Study the drawing (mm; zero at the part's minimum x, y, z) and answer. A direction names the side the tool comes from. Coordinates: 2 decimals unless noted, no trailing zeros. Write each loop counter-clockwise with the first axis right and the second up, starting at its lowest first coordinate (ties: lowest second). Pieces come first, ordered by that corner, then holes. Notation, with made-up numbers: (-10.75, 73.5) -> (9.25, 73.5) arc R23 ccw to (9.25, 94.5) -> close; hole circle Ø5 at (-27, 38). An arc over 180 degrees is marked (long way). Write item = value, one per line. Start each with the question number.
1) A tool of negligible diameter and unlimited length cuts with its end or side. For the marked faces 1 and 2, from which of +Z, -Z, +X, -X, +Y, -Y can it reach the whole face along a straight path? Write none if from no direction.
2) For a pull along Z with two mould halves and no side action, classify the marked faces 3, 4 and 5 as released by +Z, released by -Z, zero draft, split by the parting line, or undercut.
3) Flat-ended cylindrical pins translate along their axes: pin 1 Ø6.5 at (y, z) = (38.1, 11.11) entering from +X; pin 2 Ø11 at (y, z) = (25.5, 10.5) entering from +X (1 decimal); pin 3 Ø4 at (x, z) = (16.5, 7.5) entering from +Y (1 decimal); pin 4 Ø10 at (x, z) = (6.5, 12) entering from +Y. Find the tip coordinate at first contact, or state that the pin passes through.
4) Section A-A (x = 12.7) is taken. Determine the outline of the cut face in (y, z) (1 decimal).
5) Find the intervals of material crossed by line 1 along Z through (x, y) = (12.7, 2.7) (1 decimal); line 2 along X through (y, z) = (10.5, 17) (1 decimal); line 3 along Z through (x, y) = (3, 14) (1 decimal), in increasing order. Write a range as from..to.
6) Section C-C (z = 12.5) is taken. Count the separate pieces of the cut face and the enclosed holes in it, plus the area to 3 significant figures.
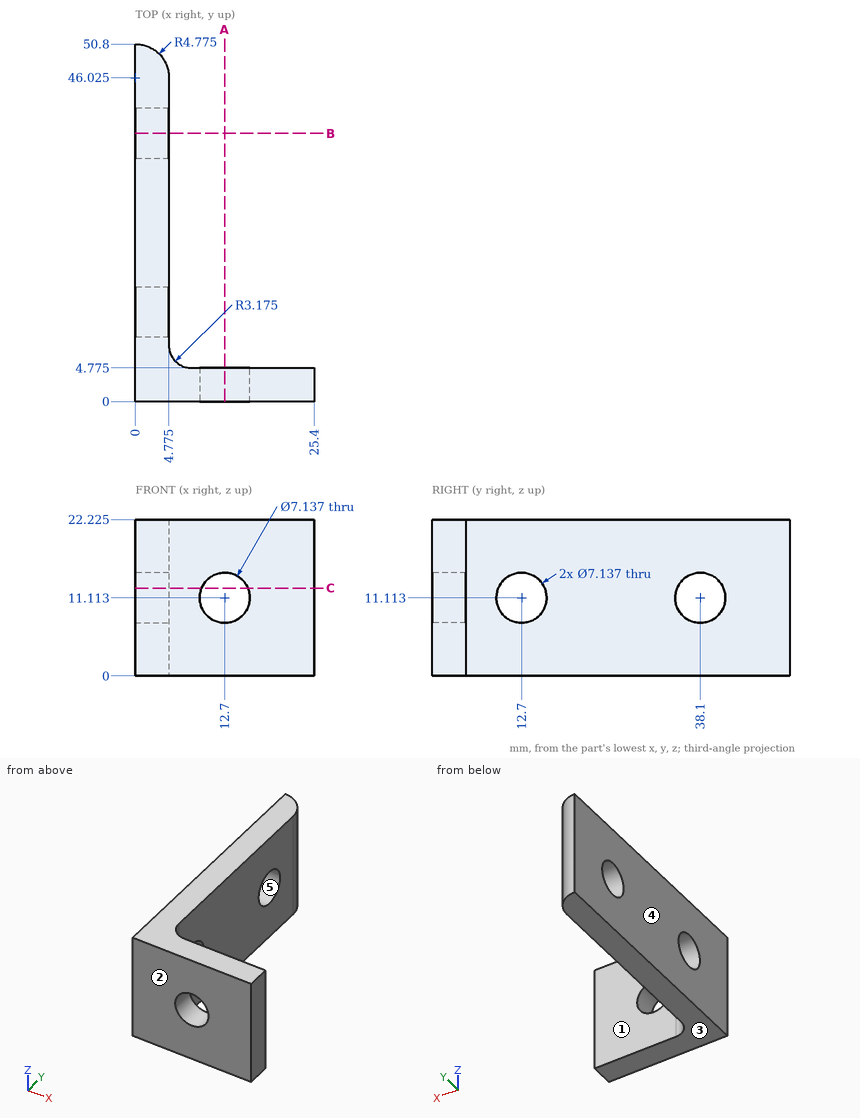
Answer key:
q1.face_1 = +Z, -Z, +X, +Y
q1.face_2 = +Z, -Z, +X, -X, -Y
q2.face_3 = released by -Z
q2.face_4 = zero draft
q2.face_5 = undercut
q3.pin_1 = through
q3.pin_2 = 4.8
q3.pin_3 = 4.8
q3.pin_4 = 50.56
q4.outline = (0, 0) -> (4.8, 0) -> (4.8, 7.5) -> (0, 7.5) -> close; (0, 14.7) -> (4.8, 14.7) -> (4.8, 22.2) -> (0, 22.2) -> close
q5.line_1 = 0..7.5, 14.7..22.2
q5.line_2 = 0..4.8
q5.line_3 = 0..7.8, 14.4..22.2
q6.separate_pieces = 4
q6.enclosed_holes = 0
q6.area = 244 mm^2
